from build123d import *

# Parameters (mm, degrees)
F1_DEPTH  = 3
F2_R      = 1.5
F2_R_2    = 2
F3_DEPTH  = 5
F4_R      = 1.5
F4_R_2    = 2
F5_DEPTH  = 5
F6_R      = 2
F7_DEPTH  = 25.4
F8_W      = 5
F8_H      = 8
F9_DEPTH  = 20
F10_R     = 2
F11_DEPTH = 25.4
F13_DEPTH = 25.4


with BuildPart() as f1:
    # F0 (on Top) → F1 (new body)
    with BuildSketch(Plane.XY):
        with BuildLine():
            Line((50, -27.5), (50, 37.5))
            Line((50, 37.5), (-50, 37.5))
            Line((-50, 37.5), (-50, -27.5))
            ThreePointArc((-50, -27.5), (-47.071068, -34.571068), (-40, -37.5))
            Line((-40, -37.5), (40, -37.5))
            ThreePointArc((40, -37.5), (47.071068, -34.571068), (50, -27.5))
        make_face()
    extrude(amount=F1_DEPTH)

    # F2 (on face) → F3 (join)
    with BuildSketch(Plane.YZ.offset(50)):
        with BuildLine():
            Line((-21.5, 13), (-21.5, 3))
            Line((-21.5, 3), (24.5, 3))
            Line((24.5, 3), (24.5, 13))
            ThreePointArc((24.5, 13), (21.571068, 20.071068), (14.5, 23))
            Line((14.5, 23), (-11.5, 23))
            ThreePointArc((-11.5, 23), (-18.571068, 20.071068), (-21.5, 13))
        make_face()
        with Locations((-17.5, 16.1)):
            Circle(F2_R, mode=Mode.SUBTRACT)
        with Locations((20.5, 16.1)):
            Circle(F2_R, mode=Mode.SUBTRACT)
        with Locations((1.5, 20)):
            Circle(F2_R_2, mode=Mode.SUBTRACT)
    extrude(amount=-F3_DEPTH)

    # F4 (on face) → F5 (join)
    with BuildSketch(Plane(origin=(-50, 0, 0), x_dir=(0, -1, 0), z_dir=(-1, 0, 0))):
        with BuildLine():
            ThreePointArc((21.5, 13), (18.571068, 20.071068), (11.5, 23))
            Line((11.5, 23), (-14.5, 23))
            ThreePointArc((-14.5, 23), (-21.571068, 20.071068), (-24.5, 13))
            Line((-24.5, 13), (-24.5, 3))
            Line((-24.5, 3), (21.5, 3))
            Line((21.5, 3), (21.5, 13))
        make_face()
        with Locations((-20.5, 16.1)):
            Circle(F4_R, mode=Mode.SUBTRACT)
        with Locations((17.5, 16.1)):
            Circle(F4_R, mode=Mode.SUBTRACT)
        with Locations((-1.5, 20)):
            Circle(F4_R_2, mode=Mode.SUBTRACT)
    extrude(amount=-F5_DEPTH)

    # F6 (on face) → F7 (cut)
    with BuildSketch(Plane.XY.offset(3)):
        with Locations((-30, 22.5)):
            Circle(F6_R)
        with Locations((-40, -27.5)):
            Circle(F6_R)
        with Locations((40, -27.5)):
            Circle(F6_R)
        with Locations((36, 22.5)):
            Circle(F6_R)
    extrude(amount=-F7_DEPTH, mode=Mode.SUBTRACT)

    # F8 (on face) → F9 (join)
    with BuildSketch(Plane.XY.offset(3)):
        with Locations((-17.5, 25.5)):
            Rectangle(F8_W, F8_H)
        with Locations((-0.5, 25.5)):
            Rectangle(F8_W, F8_H)
        with Locations((-17.5, 1.5)):
            Rectangle(F8_W, F8_H)
        with Locations((-0.5, 1.5)):
            Rectangle(F8_W, F8_H)
    extrude(amount=F9_DEPTH)

    # F10 (on face) → F11 (cut)
    with BuildSketch(Plane(origin=(-20, 0, 0), x_dir=(0, -1, 0), z_dir=(-1, 0, 0))):
        with Locations((-1.5, 20)):
            Circle(F10_R)
    extrude(amount=-F11_DEPTH, mode=Mode.SUBTRACT)

    # F12 (on face) → F13 (cut)
    with BuildSketch(Plane(origin=(-20, 0, 0), x_dir=(0, -1, 0), z_dir=(-1, 0, 0))):
        with BuildLine():
            Line((-27.5, 23), (-27.5, 20))
            ThreePointArc((-27.5, 20), (-25.5, 18), (-23.5, 20))
            Line((-23.5, 20), (-23.5, 23))
            Line((-23.5, 23), (-27.5, 23))
        make_face()
    extrude(amount=-F13_DEPTH, mode=Mode.SUBTRACT)


solid = f1.part
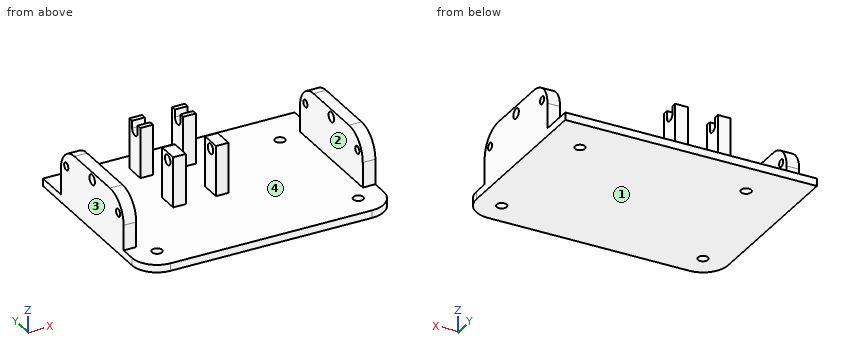
Design review of the part built by this model. Coordinates are the model's own, in mm. Face numbers are marked on the shaded views. Coordinates: 2 decimals unless noted, no trailing zeros. Write each loop counter-clockwise with the first axis right and the second up, starting at its lowest first coordinate (ties: lowest second). Pieces come first, ordered by that corner, then holes. Notation, with made-up numbers: (32, -31) - (38, -31) arc R8 cw to (38, -27) - close; hole circle Ø7 at (36, -36.5). An arc over 180 degrees is marked (long way). Use one line per item in the form item = value.
Q1. The part is to be moulded in two halves that separate along X. For the marked faces 1, 2, 3 and 4, say which applies: +X half, -X half, draft (parallel to the pull), parting line (faces both ways), or undercut.
Taken from the geometry:
face_1 = draft
face_2 = undercut
face_3 = -X half
face_4 = undercut
Q2. For probe 1 along X at (y, z) = (26.5, 7.5); probe 2 along X at (y, z) = (16, 5.75); probe 3 along Z at (x, y) = (-17.5, 1.5), list the stretches that pass through material, from the lowest coordinate up.
Taken from the geometry:
probe_1 = -20 to -15, -3 to 2
probe_2 = -50 to -45, 45 to 50
probe_3 = 0 to 18, 22 to 23
Q3. Consider section A-A (x = 0.5). Write out the cut boundary in (y, z), plus the area to 3 significant figures.
Taken from the geometry:
outline = (-37.5, 0) - (37.5, 0) - (37.5, 3) - (29.5, 3) - (29.5, 23) - (27.5, 23) - (27.5, 20) arc R2 cw to (23.5, 20) - (23.5, 23) - (21.5, 23) - (21.5, 3) - (5.5, 3) - (5.5, 23) - (-2.5, 23) - (-2.5, 3) - (-37.5, 3) - close; hole circle Ø4 at (1.5, 20)
area = 514 mm^2
Q4. Insertion check: pin 1 Ø4 at (x, z) = (-0.5, 17) entering from +Y; pin 2 Ø5.5 at (x, z) = (-1.5, 10) entering from -Y; pin 3 Ø4 at (x, z) = (47, 10) entering from -Y; pin 4 Ø3 at (x, y) = (36, 22.5) entering from -Z. Each pin has a flat end and moves straight along its axis. Give the tip position at first contact, or say it passes through.
Taken from the geometry:
pin_1 = 29.5
pin_2 = -2.5
pin_3 = -21.5
pin_4 = through
Q5. Consider section D-D (x = -30). Write out the cut boundary in (y, z), plus the area to 3 significant figures.
Taken from the geometry:
outline = (-37.5, 0) - (20.5, 0) - (20.5, 3) - (-37.5, 3) - close; (24.5, 0) - (37.5, 0) - (37.5, 3) - (24.5, 3) - close
area = 213 mm^2
Q6. Consider section C-C (z = 8). Write out the cut boundary in (x, y), plus the area to 3 significant figures.
Taken from the geometry:
outline = (-50, -21.5) - (-45, -21.5) - (-45, 24.5) - (-50, 24.5) - close; (-20, -2.5) - (-15, -2.5) - (-15, 5.5) - (-20, 5.5) - close; (-20, 21.5) - (-15, 21.5) - (-15, 29.5) - (-20, 29.5) - close; (-3, -2.5) - (2, -2.5) - (2, 5.5) - (-3, 5.5) - close; (-3, 21.5) - (2, 21.5) - (2, 29.5) - (-3, 29.5) - close; (45, -21.5) - (50, -21.5) - (50, 24.5) - (45, 24.5) - close
area = 620 mm^2
Q7. Consider section B-B (y = -17.5). Write out the cut boundary in (x, z), plus the area to 3 significant figures.
Taken from the geometry:
outline = (-50, 0) - (50, 0) - (50, 14.6) - (45, 14.6) - (45, 3) - (-45, 3) - (-45, 14.6) - (-50, 14.6) - close; (-50, 17.6) - (-45, 17.6) - (-45, 21) - (-50, 21) - close; (45, 17.6) - (50, 17.6) - (50, 21) - (45, 21) - close
area = 450 mm^2
